Here's how the part is built. I have some questions about the finished solid (model axes, mm). A direction names the side the tool comes from. Round coordinates to 2 decimals unless told otherwise and drop trailing zeros. Loops run counter-clockwise (first coordinate to the right, second up) from the corner with the lowest first, then second, coordinate; pieces in that order, holes last. Notation, with made-up numbers: (32, -10.75) - (49, -10.75) arc R15 ccw to (49, 15.25) - close; hole circle Ø9 at (74.25, -35.75). An arc over 180 degrees is marked (long way). Return JSON: item names as keys, results as strings. Group by question number.
```python
from build123d import *

# Parameters (mm, degrees)
SKETCH2_R          = 16.51
SKETCH3_R          = 20.6375
EXTRUDE1_DEPTH     = 27.686
SKETCH4_R          = 20.6375
EXTRUDE2_DEPTH     = 2.54
EXTRUDE2_TAPER     = 45
SKETCH9_R          = 16.51
SKETCH9_R_2        = 14.224
CUT_EXTRUDE4_DEPTH = 23.114
SKETCH10_R         = 16.51
SKETCH10_R_2       = 14.224
CUT_EXTRUDE5_DEPTH = 3.81
CUT_EXTRUDE5_DRAFT = 45
SKETCH11_OUTSIDE_W = 79.734
SKETCH11_OUTSIDE_H = 79.734
SKETCH11_OUTSIDE_R = 10.414
CUT_EXTRUDE6_DEPTH = 3.81
CUT_EXTRUDE6_DRAFT = -60
SHELL3_T           = 0.7366


with BuildPart() as part:
    # Sweep1: sweep along a path in Sketch1
    with BuildLine(Plane(origin=(0, 0, 0), x_dir=(0, 0, -1), z_dir=(1, 0, 0))) as sweep1_path:
        Line((51.562, 0), (-49.022, 0))
    # Sketch2 → Sweep1 (sweep)
    with BuildSketch(Plane.XY.offset(49.022)):
        Circle(SKETCH2_R)
    sweep(path=sweep1_path.line)

    # Sketch3 → Extrude1 (add)
    with BuildSketch(Plane.XY.offset(49.022)):
        Circle(SKETCH3_R)
    extrude(amount=-EXTRUDE1_DEPTH)

    # Sketch4 → Extrude2 (add)
    with BuildSketch(Plane(origin=(0, 0, 21.336), x_dir=(-1, 0, 0), z_dir=(0, 0, -1))):
        with Locations(Location((0, 0, 0), (0, 0, 180))):
            Circle(SKETCH4_R)
    extrude(amount=EXTRUDE2_DEPTH, taper=EXTRUDE2_TAPER)

    # Sketch9 → Cut-Extrude4 (cut)
    with BuildSketch(Plane(origin=(0, 0, -51.562), x_dir=(-1, 0, 0), z_dir=(0, 0, -1))):
        Circle(SKETCH9_R)
        Circle(SKETCH9_R_2, mode=Mode.SUBTRACT)
    extrude(amount=-CUT_EXTRUDE4_DEPTH, mode=Mode.SUBTRACT)


with BuildPart() as cut_extrude5_tool:
    # Sketch10 → Cut-Extrude5 (with draft: the straight prism first)
    with BuildSketch(Plane(origin=(0, 0, -28.448), x_dir=(-1, 0, 0), z_dir=(0, 0, -1))):
        Circle(SKETCH10_R)
        Circle(SKETCH10_R_2, mode=Mode.SUBTRACT)
    extrude(amount=-CUT_EXTRUDE5_DEPTH)
    # Cut-Extrude5: the draft: its side faces are tilted about the plane it starts from
    cut_extrude5_sides = [cut_extrude5_tool.faces().sort_by_distance(p)[0] for p in [
        (16.51, 0, -26.543),
        (14.224, 0, -26.543),
    ]]
    draft(cut_extrude5_sides, Plane(origin=(0, 0, -28.448), x_dir=(-1, 0, 0), z_dir=(0, 0, -1)), CUT_EXTRUDE5_DRAFT)


with BuildPart() as part_1:
    add(part.part)

    # Cut-Extrude5: cut by cut_extrude5_tool
    add(cut_extrude5_tool.part, mode=Mode.SUBTRACT)


with BuildPart() as cut_extrude6_tool:
    # Sketch11 outside → Cut-Extrude6 (with draft: the straight prism first)
    with BuildSketch(Plane(origin=(0, 0, -24.638), x_dir=(-1, 0, 0), z_dir=(0, 0, -1))):
        Rectangle(SKETCH11_OUTSIDE_W, SKETCH11_OUTSIDE_H)
        Circle(SKETCH11_OUTSIDE_R, mode=Mode.SUBTRACT)
    extrude(amount=-CUT_EXTRUDE6_DEPTH)
    # Cut-Extrude6: the draft: its side faces are tilted about the plane it starts from
    cut_extrude6_sides = [cut_extrude6_tool.faces().sort_by_distance(p)[0] for p in [
        (0, -39.867, -22.733),
        (-39.867, 0, -22.733),
        (0, 39.867, -22.733),
        (39.867, 0, -22.733),
        (10.414, 0, -22.733),
    ]]
    draft(cut_extrude6_sides, Plane(origin=(0, 0, -24.638), x_dir=(-1, 0, 0), z_dir=(0, 0, -1)), CUT_EXTRUDE6_DRAFT)


with BuildPart() as part_2:
    add(part_1.part)

    # Cut-Extrude6: cut by cut_extrude6_tool
    add(cut_extrude6_tool.part, mode=Mode.SUBTRACT)


with BuildPart() as body_2:
    # Sketch5 → Revolve1 (revolve)
    with BuildSketch(Plane(origin=(0, 0, 0), x_dir=(0, 0, -1), z_dir=(1, 0, 0)), mode=Mode.PRIVATE) as revolve1_sk:
        Polygon((11.7856, 24.384), (14.3256, 26.924), (14.3256, 50.038), (0, 50.038), (0, 0), (11.7856, 0), align=None)
    revolve(revolve1_sk.sketch.rotate(Axis((0, 50.038, 0), (0, -1, 0)), 180), axis=Axis((0, 50.038, 0), (0, -1, 0)))

    # Combine1: union part
    add(part_2.part)

    # Shell3
    shell3_openings = [body_2.faces().sort_by_distance(p)[0] for p in [
        (0, 0, -51.562),
        (0, 0, 49.022),
        (0, 50.038, 0),
    ]]
    offset(amount=SHELL3_T, openings=shell3_openings, kind=Kind.INTERSECTION)


solid = body_2.part
```
Q1. Imagine slicing it at B-B, the plane y = 34.5. List the corners of the cut face in (x, z) for me, and give its area (3 significant figures).
Q2. For faces 4 (the conical face through (-2.414, -18.389, 18.204)), 5 (the cylindrical face through (3.243, -14.605, -40.016)), 6 (the cylindrical face through (-4.474, -20.147, 35.373)), 7 (the cylindrical face through (9.17, 38.49, -11.95)), which set-ups out of +Z, -Z, +X, -X, +Y, -Y let a thin tool reach every point of the face, with its end or its side?
Q3. Imagine slicing it at A-A, the plane z = 0. List the corners of the cut face in (x, y) for me, and give its area (3 significant figures).
Q4. If we mould it in two halves opening along Z, with no side actions, what happens to faces 1 (the flat face through (15, 8, 18.796)), 2 (the flat face through (11, 14, 18.059)), 3 (the cylindrical face through (3.083, -13.886, -40.167))? For each: +Z half, -Z half, draft (parallel to the pull), parting line (faces both ways), or undercut.
Q5. Imagine slicing it at C-C, the plane z = 17. List the corners of the cut face in (x, y) for me.
Q6. Will these pins go through, and if not, where does the flat tip stop? pin 1 Ø8 at (y, z) = (-6, -10) entering from +X; pin 2 Ø5 at (y, z) = (13, 33) entering from +X; pin 3 Ø2 at (x, z) = (-8, -37.5) entering from +Y; pin 4 Ø3 at (x, y) = (-8.5, -0.5) entering from +Z.
Q7. Please list where these lines run through material, in increasing order: line 1 (X direction, y = 35.5, z = 0); line 2 (Y direction, x = 0, z = -45.75); line 3 (Y direction, x = 14.5, z = -3).
Q8. Imagine slicing it at D-D, the plane x = 7. Give the number of separate pieces and of enclosed holes in the cut face, and give its area (3 significant figures).
Output values:
{
 "1": {"outline": "circle Ø30.12 at (0, 0); hole circle Ø28.65 at (0, 0)", "area": "68.0 mm^2"},
 "2": {"face 4": "none", "face 5": "-Z", "face 6": "+Z", "face 7": "+Y"},
 "3": {"outline": "(-15.06, 26.62) - (-12.52, 24.08) - (-12.52, 11.86) arc R17.25 ccw (long way) to (12.52, 11.86) - (12.52, 24.08) - (15.06, 26.62) - (15.06, 50.04) - (14.33, 50.04) - (14.33, 26.92) - (11.79, 24.38) - (11.79, 11.56) arc R16.51 cw (long way) to (-11.79, 11.56) - (-11.79, 24.38) - (-14.33, 26.92) - (-14.33, 50.04) - (-15.06, 50.04) - close", "area": "116 mm^2"},
 "4": {"face 1": "+Z half", "face 2": "undercut", "face 3": "draft"},
 "5": {"outline": "circle Ø34.49 at (0, 0); hole circle Ø33.02 at (0, 0)"},
 "6": {"pin 1": "stops at x = 17.13", "pin 2": "stops at x = 18.62", "pin 3": "stops at y = 13.22", "pin 4": "passes through"},
 "7": {"line 1": "x = -15.06 to -14.33, 14.33 to 15.06", "line 2": "y = -14.96 to -14.22, 14.22 to 14.96", "line 3": "y = -9.34 to -7.89, 7.89 to 9.34, 26.36 to 50.04"},
 "8": {"separate pieces": "3", "enclosed holes": "0", "area": "221 mm^2"}
}
